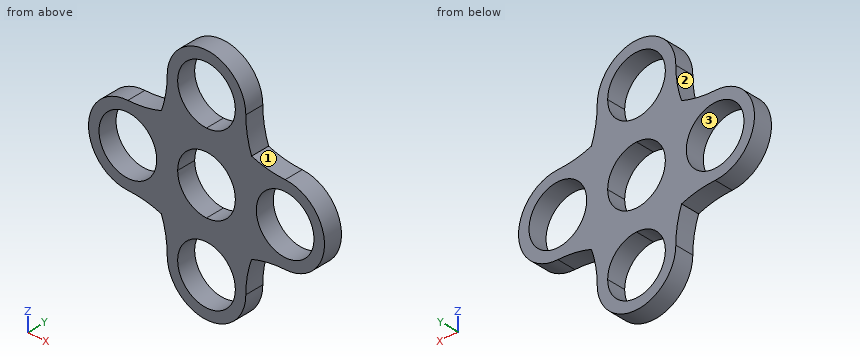
from build123d import *

# Parameters (mm, degrees)
F0_R     = 11
F1_DEPTH = 7


with BuildPart() as f1:
    # F0 (on Front) → F1 (new body)
    with BuildSketch(Plane.XZ):
        with BuildLine():
            ThreePointArc((30, -15), (45, 0), (30, 15))
            ThreePointArc((30, 15), (23.504809, 15.553158), (17.196699, 17.196699))
            ThreePointArc((17.196699, 17.196699), (15.553158, 23.504809), (15, 30))
            ThreePointArc((15, 30), (0, 45), (-15, 30))
            ThreePointArc((-15, 30), (-15.553158, 23.504809), (-17.196699, 17.196699))
            ThreePointArc((-17.196699, 17.196699), (-23.504809, 15.553158), (-30, 15))
            ThreePointArc((-30, 15), (-45, 0), (-30, -15))
            ThreePointArc((-30, -15), (-23.504809, -15.553158), (-17.196699, -17.196699))
            ThreePointArc((-17.196699, -17.196699), (-15.553158, -23.504809), (-15, -30))
            ThreePointArc((-15, -30), (0, -45), (15, -30))
            ThreePointArc((15, -30), (15.553158, -23.504809), (17.196699, -17.196699))
            ThreePointArc((17.196699, -17.196699), (23.504809, -15.553158), (30, -15))
        make_face()
        with BuildLine():
            ThreePointArc((11, -30), (-7.778175, -37.778175), (0, -19))
            ThreePointArc((0, -19), (7.778175, -22.221825), (11, -30))
        make_face(mode=Mode.SUBTRACT)
        with Locations((-30, 0)):
            Circle(F0_R, mode=Mode.SUBTRACT)
        with BuildLine():
            ThreePointArc((11, 0), (7.778175, -7.778175), (0, -11))
            ThreePointArc((0, -11), (-7.778175, -7.778175), (-11, 0))
            ThreePointArc((-11, 0), (-7.778175, 7.778175), (0, 11))
            ThreePointArc((0, 11), (7.778175, 7.778175), (11, 0))
        make_face(mode=Mode.SUBTRACT)
        with BuildLine():
            ThreePointArc((41, 0), (30, -11), (19, 0))
            ThreePointArc((19, 0), (30, 11), (41, 0))
        make_face(mode=Mode.SUBTRACT)
        with BuildLine():
            ThreePointArc((11, 30), (7.778175, 22.221825), (0, 19))
            ThreePointArc((0, 19), (-7.778175, 37.778175), (11, 30))
        make_face(mode=Mode.SUBTRACT)
    extrude(amount=F1_DEPTH)


solid = f1.part
Geometry check sheet. Reference: the model listing, model coordinates, mm. Face numbers are marked on the shaded views. Give positions to 0.01 mm unless a question says otherwise; leave off trailing zeros. Order: outer loops, then holes, each group sorted by start corner. A loop starts at its lowest first (then second) coordinate and runs counter-clockwise, first axis right, second up. Notation, with made-up numbers: (-16, 19) - (21, 19) arc R22 cw to (21, 33) - close; hole circle Ø4 at (87.5, 62). An arc over 180 degrees is marked (long way). Answer as a JSON object with one key per item and string values.
(1) Material ranges on line 1 (X direction, y = -0.5, z = -0.5); line 2 (Z direction, x = -30, y = -5); line 3 (X direction, y = -5.75, z = -4.5), recorded low to high.
Report:
{"line 1": "-44.99 to -40.99, -19.01 to -10.99, 10.99 to 19.01, 40.99 to 44.99", "line 2": "-15 to -11, 11 to 15", "line 3": "-44.31 to -40.04, -19.96 to -10.04, 10.04 to 19.96, 40.04 to 44.31"}
(2) Cross-section at B-B (x = -34.5). Record the cut outline in (y, z), then the cut area to 3 significant figures.
Report:
{"outline": "(-7, -14.31) - (0, -14.31) - (0, -10.04) - (-7, -10.04) - close; (-7, 10.04) - (0, 10.04) - (0, 14.31) - (-7, 14.31) - close", "area": "59.8 mm^2"}
(3) Cross-section at D-D (x = -13). Record the cut outline in (y, z).
Report:
{"outline": "(-7, -37.48) - (0, -37.48) - (0, 37.48) - (-7, 37.48) - close"}
(4) Cross-section at A-A (y = -4.5). Record the cut outline in (x, z).
Report:
{"outline": "(-30, -15) arc R38.41 cw to (-17.2, -17.2) arc R38.41 cw to (-15, -30) arc R15 ccw to (15, -30) arc R38.41 cw to (17.2, -17.2) arc R38.41 cw to (30, -15) arc R15 ccw to (30, 15) arc R38.41 cw to (17.2, 17.2) arc R38.41 cw to (15, 30) arc R15 ccw to (-15, 30) arc R38.41 cw to (-17.2, 17.2) arc R38.41 cw to (-30, 15) arc R15 ccw to start; hole circle Ø22 at (-30, 0); hole (-11, 0) arc R11 ccw to (0, -11) arc R11 ccw to (11, 0) arc R11 ccw to (0, 11) arc R11 ccw to start; hole (0, -19) arc R11 ccw (long way) to (11, -30) arc R11 ccw to start; hole (0, 19) arc R11 ccw to (11, 30) arc R11 ccw (long way) to start; hole circle Ø22 at (30, 0)"}
(5) Cross-section at C-C (z = -21). Record the cut outline in (x, y).
Report:
{"outline": "(-16.07, -7) - (-6.32, -7) - (-6.32, 0) - (-16.07, 0) - close; (6.32, -7) - (16.07, -7) - (16.07, 0) - (6.32, 0) - close"}
(6) Draft check along X on the marked faces 1, 2 and 3. Enter one of: released by +X, released by -X, zero draft, split by the parting line, or undercut.
Report:
{"face 1": "released by +X", "face 2": "released by -X", "face 3": "undercut"}
(7) Depth check by flat-ended pin: pin 1 Ø1.5 at (x, y) = (20, -2) entering from -Z (3 decimals). Enter the tip coordinate at first touch or a pass-through.
Report:
{"pin 1": "z = -16.535"}
